Can you work these out from the model? Positions are in its coordinate system, mm. A direction names the side the tool comes from. Coordinates: 2 decimals unless noted, no trailing zeros. Write each loop counter-clockwise with the first axis right and the second up, starting at its lowest first coordinate (ties: lowest second). Pieces come first, ordered by that corner, then holes. Notation, with made-up numbers: M -7.5,-30 L 11.5,-30 A30 ccw 11.5,0 Z; hole C 1,69.25 d11. An arc over 180 degrees is marked long. Answer as a JSON object with one key per item and string values. Group by question number.
from build123d import *

# Parameters (mm, degrees)
F0_W     = 6.35
F0_H     = 6.35
F1_DEPTH = 18.15
F2_D     = 3
F2_DEPTH = 7
F2_TIP   = 0.9012909285
F4_D     = 3
F4_DEPTH = 7
F4_TIP   = 0.9012909285


with BuildPart() as f1:
    # F0 (on Top) → F1 (new body)
    with BuildSketch(Plane.XY):
        Rectangle(F0_W, F0_H)
    extrude(amount=F1_DEPTH)

    # F2
    with Locations(Plane(origin=(0, 0, 0), x_dir=(1, 0, 0), z_dir=(0, 0, -1))):
        with Locations((0, 0)):
            Hole(F2_D / 2, depth=F2_DEPTH)
            with Locations((0, 0, -(F2_DEPTH + F2_TIP / 2))):  # 118° drill point
                Cone(0, F2_D / 2, F2_TIP, mode=Mode.SUBTRACT)

    # F4
    with Locations(Plane.XY.offset(18.15)):
        with Locations((0, 0)):
            Hole(F4_D / 2, depth=F4_DEPTH)
            with Locations((0, 0, -(F4_DEPTH + F4_TIP / 2))):  # 118° drill point
                Cone(0, F4_D / 2, F4_TIP, mode=Mode.SUBTRACT)


solid = f1.part
Q1. Will these pins go through, and if not, where does the flat tip stop? pin 1 (2.5 mm diameter, centred on x = 0, y = 0, fed in from +Z); pin 2 (1.8 mm diameter, centred on x = 0, y = 0, fed in from +Z).
Q2. We'd pull the mould along Y, two halves only. Please class faces 1 (the flat face through (0, 3.175, 9)), 2 (the flat face through (3.175, 0, 9)), 3 (the cylindrical face through (1.5, 0.07, 14.6)): pulls with the +Y half, pulls with the -Y half, needs draft (parallel to the pull), parting line crosses it, or undercut.
Q3. If we section it at A-A on z = 12: List the corners of the cut face in (x, y) for me (3 decimals), and give its area (3 significant figures).
Q4. Please list where these lines run through material, in increasing order: L1, parallel to X at y = 0, z = 16 (3 decimals); L2, parallel to X at y = -1.25, z = 12.25 (3 decimals).
Q5. On a 3-axis mill with a long thin cutter (end or side, diameter ignored), from which of +Z, -Z, +X, -X, +Y, -Y can I reach the whole of each face in a straight line? I mean faces 4 (the cylindrical face through (1.5, -0.07, 3.55)), 5 (the conical face through (-0.056, -0.254, 10.405)). Say none if no direction works.
Reply:
{
 "1": {"pin 1": "z = 11", "pin 2": "z = 10.79"},
 "2": {"face 1": "pulls with the +Y half", "face 2": "needs draft", "face 3": "undercut"},
 "3": {"outline": "M -3.175,-3.175 L 3.175,-3.175 L 3.175,3.175 L -3.175,3.175 Z; hole C 0,0 d3", "area": "33.3 mm^2"},
 "4": {"L1": "-3.175 to -1.5, 1.5 to 3.175", "L2": "-3.175 to -0.829, 0.829 to 3.175"},
 "5": {"face 4": "-Z", "face 5": "+Z"}
}
